For this review, take the finished solid that the model builds, in its own axes (mm). A direction names the side the tool comes from. Round coordinates to 2 decimals unless told otherwise and drop trailing zeros. Loops run counter-clockwise (first coordinate to the right, second up) from the corner with the lowest first, then second, coordinate; pieces in that order, holes last. Notation, with made-up numbers: (80.25, 80) -> (104.25, 80) arc R15 cw to (104.25, 104) -> close; hole circle Ø4 at (36.5, 26). An arc over 180 degrees is marked (long way). One line per question, with ' | ' between items. Start each with the question number.
1. Draft analysis for pull direction Z (two halves, no side actions). For faces 1 (the face through (9.139, 14.334, 1.521)), 2 (the face through (-6, 13, 3)), 3 (the face through (2.86, 0.9, 6)), state which applies: pulls with the +Z half, pulls with the -Z half, needs draft (parallel to the pull), parting line crosses it, or undercut.
2. Consider section A-A (z = 7). Write out the cut boundary in (x, y).
3. For faces 4 (the face through (-0.338, 2.578, 8.372)), 5 (the face through (6, 13, 8)), 6 (the face through (9.139, 14.334, 13.45)), list the 3-axis set-ups (+Z, -Z, +X, -X, +Y, -Y) from which the entire face can be reached by the end or side of a thin tool; tool diameter is ignored.
4. For pin 1 Ø4 at (y, z) = (8.5, 15.5) entering from +X; pin 2 Ø17 at (x, y) = (0.5, 0.5) entering from +Z; pin 3 Ø3 at (y, z) = (-5.5, 11) entering from +X, all flat-tipped, find the tip position at first contact; note any pin that passes through.
5. Wall thickness on line 1 along Y through (x, z) = (0, 8.3); line 2 along Y through (x, z) = (0, 7.5); line 3 along Z through (x, y) = (-13.5, -5): over which ranges is each line inside the solid? List them lowest first.
```python
from build123d import *


with BuildPart() as f1:
    # F0 (on Front) → F1 (revolve)
    with BuildSketch(Plane.XZ):
        with BuildLine():
            ThreePointArc((14.677176, 19.761905), (7.715167, 16.220257), (0, 15))
            Line((0, 15), (0, 13))
            Line((0, 13), (2.6, 10.4))
            Line((2.6, 10.4), (2.6, 6.4))
            Line((2.6, 6.4), (9, 0))
            Line((9, 0), (17, 0))
            Line((17, 0), (17, 3))
            Line((17, 3), (14, 3))
            Line((14, 3), (14, 8))
            Line((14, 8), (17, 8))
            Line((17, 8), (17, 18.75))
            ThreePointArc((17, 18.75), (16.633883, 19.633883), (15.75, 20))
            Line((15.75, 20), (15.411035, 20))
            ThreePointArc((15.411035, 20), (15.025277, 19.938987), (14.677176, 19.761905))
        make_face()
    revolve(axis=Axis((0, 0, 7.5), (0, 0, 1)))


solid = f1.part
```
Answer block:
1) face 1: needs draft | face 2: undercut | face 3: pulls with the -Z half
2) outline: circle Ø28 at (0, 0); hole circle Ø5.2 at (0, 0)
3) face 4: -Z | face 5: none | face 6: +Z, -Z
4) pin 1: stops at x = 15.71 | pin 2: stops at z = 16.76 | pin 3: stops at x = 16.52
5) line 1: y = -17 to -2.6, 2.6 to 17 | line 2: y = -14 to -2.6, 2.6 to 14 | line 3: z = 0 to 3, 8 to 19.56
